```python
from build123d import *

# Parameters (mm, degrees)
SZKIC1_R                    = 10
DODANIE_WYCI_GNI_CIE1_DEPTH = 2


with BuildPart() as part:
    # Szkic1 → Dodanie-wyciągnięcie1 (new body)
    with BuildSketch(Plane(origin=(0, 0, 0), x_dir=(1, 0, 0), z_dir=(0, 1, 0))):
        with BuildLine():
            add(Edge.make_bspline(
                [(25.724787771, -25.724787771), (50, -16.985711369), (50, 0)],
                knots=[5.252808481, 5.252808481, 5.252808481, 6.283185307, 6.283185307, 6.283185307], degree=2, weights=[1, 0.870199907, 1]))
            Line((50, 0), (30, 0))
            add(Edge.make_bspline(
                [(30, 0), (30, 13.849198247), (25.724787771, 25.724787771)],
                knots=[1.570796327, 1.570796327, 1.570796327, 2.111215827, 2.111215827, 2.111215827], degree=2, weights=[1, 0.963714928, 1]))
            add(Edge.make_bspline(
                [(25.724787771, 25.724787771), (23.68927397, 31.378992774), (20.843852414, 35.960387795)],
                knots=[2.111215827, 2.111215827, 2.111215827, 2.373457716, 2.373457716, 2.373457716], degree=2, weights=[1, 0.991415958, 1]))
            Line((20.843852414, 35.960387795), (7.507535684, 33.029118956))
            add(Edge.make_bspline(
                [(7.507535684, 33.029118956), (5.218865934, 46.034514162), (1.811566447, 49.17271271)],
                knots=[5.433983203, 5.433983203, 5.433983203, 6.101022879, 6.101022879, 6.101022879], degree=2, weights=[1, 0.944895907, 1]))
            add(Edge.make_bspline(
                [(1.811566447, 49.17271271), (0.913339162, 50), (0, 50)],
                knots=[6.101022879, 6.101022879, 6.101022879, 6.283185307, 6.283185307, 6.283185307], degree=2, weights=[1, 0.995854973, 1]))
            add(Edge.make_bspline(
                [(0, 50), (-0.913339162, 50), (-1.811566447, 49.17271271)],
                knots=[0, 0, 0, 0.182162428, 0.182162428, 0.182162428], degree=2, weights=[1, 0.995854973, 1]))
            add(Edge.make_bspline(
                [(-1.811566447, 49.17271271), (-5.218865934, 46.034514162), (-7.507535684, 33.029118956)],
                knots=[0.182162428, 0.182162428, 0.182162428, 0.849202104, 0.849202104, 0.849202104], degree=2, weights=[1, 0.944895907, 1]))
            Line((-7.507535684, 33.029118956), (-20.843852414, 35.960387795))
            add(Edge.make_bspline(
                [(-20.843852414, 35.960387795), (-23.68927397, 31.378992774), (-25.724787771, 25.724787771)],
                knots=[3.909727591, 3.909727591, 3.909727591, 4.17196948, 4.17196948, 4.17196948], degree=2, weights=[1, 0.991415958, 1]))
            add(Edge.make_bspline(
                [(-25.724787771, 25.724787771), (-50, 16.985711369), (-50, 0)],
                knots=[2.111215827, 2.111215827, 2.111215827, 3.141592654, 3.141592654, 3.141592654], degree=2, weights=[1, 0.870199907, 1]))
            Line((-50, 0), (-30, 0))
            add(Edge.make_bspline(
                [(-30, 9.5e-08), (-30.000000016, -13.849198204), (-25.724787771, -25.724787771)],
                knots=[4.712388978, 4.712388978, 4.712388978, 5.252808481, 5.252808481, 5.252808481], degree=2, weights=[1, 0.963714928, 1]))
            Line((-25.724787771, -25.724787771), (-29.607826273, -37.88667404))
            Line((-29.607826273, -37.88667404), (-20.843852414, -35.960387795))
            add(Edge.make_bspline(
                [(-20.843852414, -35.960387795), (-12.774167321, -48.953336072), (-1.56928672, -49.931545896)],
                knots=[5.51505037, 5.51505037, 5.51505037, 6.230851865, 6.230851865, 6.230851865], degree=2, weights=[1, 0.936634273, 1]))
            add(Edge.make_bspline(
                [(-1.56928672, -49.931545896), (-0.785180849, -50), (0, -50)],
                knots=[6.230851865, 6.230851865, 6.230851865, 6.283185307, 6.283185307, 6.283185307], degree=2, weights=[1, 0.999657671, 1]))
            add(Edge.make_bspline(
                [(0, -50), (0.785180849, -50), (1.56928672, -49.931545896)],
                knots=[0, 0, 0, 0.052333442, 0.052333442, 0.052333442], degree=2, weights=[1, 0.999657671, 1]))
            add(Edge.make_bspline(
                [(1.56928672, -49.931545896), (12.774167321, -48.953336072), (20.843852414, -35.960387795)],
                knots=[0.052333442, 0.052333442, 0.052333442, 0.768134938, 0.768134938, 0.768134938], degree=2, weights=[1, 0.936634273, 1]))
            Line((20.843852414, -35.960387795), (29.607826273, -37.88667404))
            Line((29.607826273, -37.88667404), (25.724787771, -25.724787771))
        make_face()
        with Locations(Location((0, 0, 0), (0, 0, 270))):
            Circle(SZKIC1_R, mode=Mode.SUBTRACT)
    extrude(amount=DODANIE_WYCI_GNI_CIE1_DEPTH)


solid = part.part
```
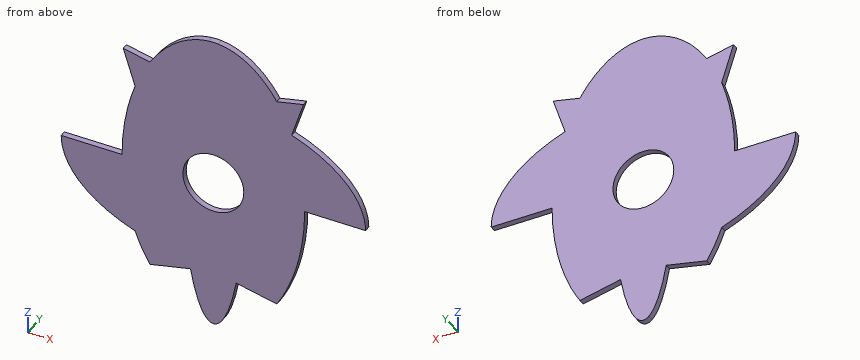
Part model, mm, in its own coordinate system. Round coordinates to 2 decimals unless told otherwise and drop trailing zeros. Order: outer loops, then holes, each group sorted by start corner. A loop starts at its lowest first (then second) coordinate and runs counter-clockwise, first axis right, second up. Notation, with made-up numbers: M 23.5,-29 L 68.5,-29 A13 cw 68.5,-24 Z; hole C 19.5,41.5 d9. An arc over 180 degrees is marked long. Answer in a Markdown table with one row per item. Add a question column.
Q1. Wall check: L1, parallel to Z at x = 9, y = 0.6; L2, parallel to Z at x = -11.5, y = 0.6; L3, parallel to Z at x = -24, y = 1.15. Give the ranges that are in metal, low to high. Write a range as from..to.
Q2. Pin check, flat tips, straight feed: pin 1 (0.6 mm diameter, centred on x = 36, y = 1, fed in from -Z); pin 2 (1 mm diameter, centred on y = 1, z = 1, fed in from -X). Stop position of each tip, or through.
Q3. Cut at A-A on z = 33. Give the cut face in (x, y), and give its area (3 significant figures).
Established:
| question | item | result |
|---|---|---|
| 1 | L1 | z = -33.36..-4.36, 4.36..47.7 |
| 1 | L2 | z = -33.91..46.18 |
| 1 | L3 | z = -30..36.65 |
| 2 | pin 1 | stops at z = 0 |
| 2 | pin 2 | stops at x = -30 |
| 3 | outline | M -28.05,0 L 28.05,0 L 28.05,2 L -28.05,2 Z |
| 3 | area | 112 mm2 |
